Answer from the drawing. Dimensions are ordinates in mm from the lowest x, y and z of the part. Give positions to 0.01 mm unless a question says otherwise; leave off trailing zeros. Loops run counter-clockwise (first coordinate to the right, second up) from the corner with the lowest first, then second, coordinate; pieces in that order, holes last. Notation, with made-up numbers: M -8,29 L 15,29 A28 cw 15,68 Z; hole C 50,-31 d2. An arc over 180 degrees is marked long. Return JSON: item names as keys, results as strings. Group by question number.
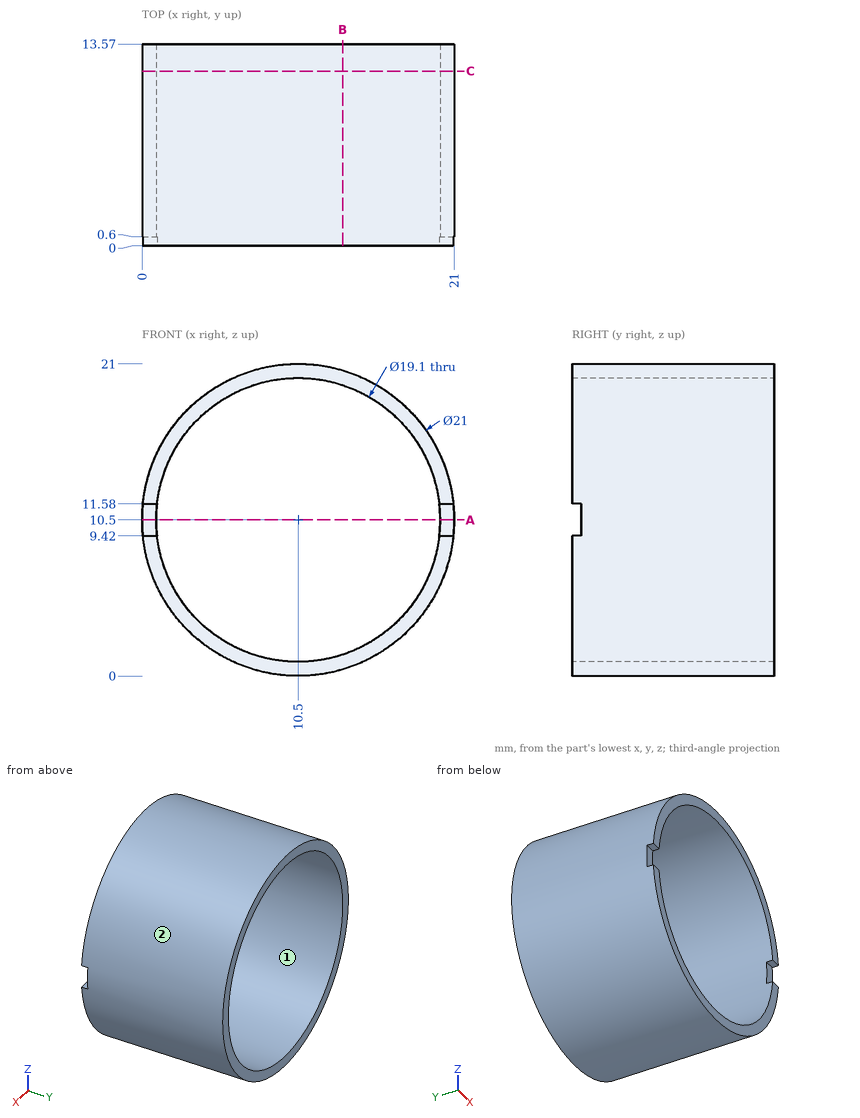
1. Find section A-A (z = 10.5). Write down the section's boundary in (x, y).
2. Find section C-C (y = 11.75). Write down the section's boundary in (x, z).
3. Straight lines are drawn through the part: line 1 along X through (y, z) = (9, 10.5); line 2 along X through (y, z) = (9.25, 9.25); line 3 along Z through (x, y) = (4.25, 1.25). For each, find the intervals that lie inside material, in ascending order.
4. Find section B-B (x = 13.5). Write down the section's boundary in (y, z).
5. Flat-ended cylindrical pins translate along their axes: P1, Ø1, axis at x = 8, y = 11, coming from the +Z side; P2, Ø0.7, axis at x = 1, y = 0.5, coming from the -Z side. Find the tip coordinate at first contact, or state that the pin passes through.
6. The mould has two halves that part along X. Classify the marked faces 1 and 2: +X half, -X half, draft (parallel to the pull), parting line (faces both ways), or undercut.
Result:
{
 "1": {"outline": "M 0,0.6 L 0.95,0.6 L 0.95,13.57 L 0,13.57 Z; M 20.05,0.6 L 21,0.6 L 21,13.57 L 20.05,13.57 Z"},
 "2": {"outline": "C 10.5,10.5 d21; hole C 10.5,10.5 d19.1"},
 "3": {"line 1": "x = 0 to 0.95, 20.05 to 21", "line 2": "x = 0.07 to 1.03, 19.97 to 20.93", "line 3": "z = 2.06 to 3.28, 17.72 to 18.94"},
 "4": {"outline": "M 0,0.44 L 13.57,0.44 L 13.57,1.43 L 0,1.43 Z; M 0,19.57 L 13.57,19.57 L 13.57,20.56 L 0,20.56 Z"},
 "5": {"P1": "stops at z = 20.81", "P2": "stops at z = 5.35"},
 "6": {"face 1": "undercut", "face 2": "parting line"}
}
